```python
from build123d import *

# Parameters (mm, degrees)
BOSS_EXTRUDE1_DEPTH      = 15
BOSS_EXTRUDE1_DEPTH_BACK = 11
BOSS_EXTRUDE2_DEPTH      = 9
FILLET1_START            = -60
FILLET1_DEPTH            = 60
FILLET2_START            = -60
FILLET2_DEPTH            = 60
SKETCH2_R                = 4.5
CUT_EXTRUDE1_DEPTH       = 88
FILLET3_R                = 2
FILLET4_R                = 2


with BuildPart() as part:
    # Sketch1 → Boss-Extrude1 (new, two sides: drawn at the far end of the back side and taken through both)
    with BuildSketch(Plane.XY.offset(-BOSS_EXTRUDE1_DEPTH_BACK)):
        with BuildLine():
            Line((-27, 0), (-36, 0))
            ThreePointArc((-36, 0), (0, -36), (36, 0))
            Line((36, 0), (27, 0))
            ThreePointArc((27, 0), (0, -27), (-27, 0))
        make_face()
    extrude(amount=BOSS_EXTRUDE1_DEPTH + BOSS_EXTRUDE1_DEPTH_BACK)

    # Sketch1<3> → Boss-Extrude2 (add, symmetric)
    with BuildSketch(Plane.XY):
        with BuildLine():
            ThreePointArc((-36, 0), (0, -36), (36, 0))
            Line((36, 0), (47, 0))
            Line((47, 0), (47, -40))
            Line((47, -40), (22, -60))
            Line((22, -60), (-22, -60))
            Line((-22, -60), (-47, -40))
            Line((-47, -40), (-47, 0))
            Line((-47, 0), (-36, 0))
        make_face()
    extrude(amount=BOSS_EXTRUDE2_DEPTH, both=True)

    # Fillet1: read off the stored shape, not the designer's step
    # Fillet1 outline → Fillet1 (cut)
    with BuildSketch(Plane(origin=(0, 0, 0), x_dir=(1, 0, 0), z_dir=(0, 1, 0)).offset(FILLET1_START)):
        with BuildLine():
            Line((47, 9), (38, 9))
            ThreePointArc((38, 9), (44.363961031, 6.363961031), (47, 0))
            Line((47, 0), (47, 9))
        make_face()
        with BuildLine():
            Line((47, -9), (47, 0))
            ThreePointArc((47, 0), (44.363961031, -6.363961031), (38, -9))
            Line((38, -9), (47, -9))
        make_face()
    extrude(amount=FILLET1_DEPTH, mode=Mode.SUBTRACT)

    # Fillet2: read off the stored shape, not the designer's step
    # Fillet2 outline → Fillet2 (cut)
    with BuildSketch(Plane(origin=(0, 0, 0), x_dir=(1, 0, 0), z_dir=(0, 1, 0)).offset(FILLET2_START)):
        with BuildLine():
            Line((-47, -9), (-38, -9))
            ThreePointArc((-38, -9), (-44.363961031, -6.363961031), (-47, 0))
            Line((-47, 0), (-47, -9))
        make_face()
        with BuildLine():
            Line((-47, 9), (-47, 0))
            ThreePointArc((-47, 0), (-44.363961031, 6.363961031), (-38, 9))
            Line((-38, 9), (-47, 9))
        make_face()
    extrude(amount=FILLET2_DEPTH, mode=Mode.SUBTRACT)

    # Sketch2 → Cut-Extrude1 (cut)
    with BuildSketch(Plane(origin=(0, 0, 0), x_dir=(1, 0, 0), z_dir=(0, 1, 0))):
        with Locations(Location((38, 0, 0), (0, 0, 270))):
            Circle(SKETCH2_R)
        with Locations(Location((-38, 0, 0), (0, 0, 180))):
            Circle(SKETCH2_R)
    extrude(amount=-CUT_EXTRUDE1_DEPTH, mode=Mode.SUBTRACT)

    # Fillet3
    fillet3_edges = [part.edges().sort_by_distance(p)[0] for p in [
        (0, -36, 15),
        (0, -36, -9),
        (0, -36, 9),
    ]]
    fillet(fillet3_edges, radius=FILLET3_R - 0.0001)  # a hair under: the kernel refuses the full size

    # Fillet4
    fillet4_edges = [part.edges().sort_by_distance(p)[0] for p in [
        (0, -27, 15),
        (0, -27, -11),
    ]]
    fillet(fillet4_edges, radius=FILLET4_R)


solid = part.part
```
CAD build for the part. Positions are in the model's coordinates, mm. A direction names the side the tool comes from. Give positions to 0.01 mm unless a question says otherwise; leave off trailing zeros. Loops run counter-clockwise (first coordinate to the right, second up) from the corner with the lowest first, then second, coordinate; pieces in that order, holes last. Notation, with made-up numbers: (86, 11.25) - (104, 11.25) arc R18 ccw to (104, 37.25) - close; hole circle Ø9 at (6, 62.25). An arc over 180 degrees is marked (long way). Put each result on its own line as item: value.
Q1. Slice it at C-C (y = -14.5). Give the number of separate pieces and of enclosed holes in the cut face, plus the area to 3 significant figures.
Filled in:
separate pieces: 2
enclosed holes: 2
area: 836 mm²
Q2. Flat gauge pins, fed straight in: pin 1 (7 mm diameter, centred on x = -38, z = 0, fed in from +Y); pin 2 (4 mm diameter, centred on y = -38.5, z = -4, fed in from +X); pin 3 (5 mm diameter, centred on y = -34, z = -5.5, fed in from +X); pin 4 (1.5 mm diameter, centred on y = -29, z = 6, fed in from -X). Where does each tip first touch, or does it go through?
Filled in:
pin 1: passes through
pin 2: stops at x = 46.77
pin 3: stops at x = 46.49
pin 4: stops at x = -45.31
Q3. Probe line 1 along Z through (x, y) = (-38, -31.5); line 2 along X through (y, z) = (-56, -0.25); line 3 along Y through (x, z) = (1, 0.75). List the from-to ranges inside material, lowest first.
Filled in:
line 1: z = -9 to -4.5, 4.5 to 9
line 2: x = -27 to 27
line 3: y = -60 to -26.98
Q4. Slice it at D-D (z = -2.5). Give the cut face in (x, y).
Filled in:
outline: (-46.65, -40.28) - (-41.74, -44.21) - (-41.74, 0) - (-46.65, 0) - close; (-34.26, -50.19) - (-22, -60) - (22, -60) - (34.26, -50.19) - (34.26, 0) - (27, 0) arc R27 cw to (-27, 0) - (-34.26, 0) - close; (41.74, -44.21) - (46.65, -40.28) - (46.65, 0) - (41.74, 0) - close
Q5. Tool access for faces 4 (the face through (-32, -52, 0)), 5 (the face through (1, -43, -9)), 6 (the face through (1, -43, 9)): list every direction of +Z, -Z, +X, -X, +Y, -Y with a clear straight run to the whole face (end or side of a thin tool).
Filled in:
face 4: +Z, -Z, -X, -Y
face 5: -Z, -Y
face 6: +Z, -Y
Q6. Slice it at A-A (z = 2.25). Give the cut face in (x, y), plus the area to 3 significant figures.
Filled in:
outline: (-46.71, -40.23) - (-41.9, -44.08) - (-41.9, 0) - (-46.71, 0) - close; (-34.1, -50.32) - (-22, -60) - (22, -60) - (34.1, -50.32) - (34.1, 0) - (27, 0) arc R27 cw to (-27, 0) - (-34.1, 0) - close; (41.9, -44.08) - (46.71, -40.23) - (46.71, 0) - (41.9, 0) - close
area: 3,240 mm²
Q7. Mould opens along X. For faces 1 (the face through (32, -52, 0)), 2 (the face through (33, 0, 2)), 3 (the face through (0.594, -26.993, 1.846)) say: pulls with the +X half, pulls with the -X half, needs draft (parallel to the pull), parting line crosses it, or undercut.
Filled in:
face 1: pulls with the +X half
face 2: needs draft
face 3: undercut
